```python
from build123d import *

# Parameters (mm, degrees)
SKETCH1_W              = 165.1
SKETCH1_H              = 114.3
BOSS_EXTRUDE1_DEPTH    = 6.35
F_10_24_TAPPED_HOLE2_D = 3.7973
F_6_32_TAPPED_HOLE2_D  = 2.7051
CUT_EXTRUDE10_DEPTH    = 101.602919938
F_6_32_TAPPED_HOLE1_D  = 2.7051
SKETCH24_W             = 107.95
SKETCH24_H             = 71.12
CUT_EXTRUDE11_DEPTH    = 101.602919938
FILLET1_R              = 3.175


with BuildPart() as part:
    # Sketch1 → Boss-Extrude1 (new body)
    with BuildSketch(Plane(origin=(0, 0, 0), x_dir=(1, 0, 0), z_dir=(0, 1, 0))):
        Rectangle(SKETCH1_W, SKETCH1_H)
    extrude(amount=BOSS_EXTRUDE1_DEPTH)

    # #10-24 Tapped Hole2 (through all)
    with Locations(Plane(origin=(0, 6.35, 0), x_dir=(-1, 0, 0), z_dir=(0, 1, 0))):
        with Locations((73.025, -47.625), (73.025, 47.625), (-73.025, -47.625), (-73.025, 47.625)):
            Hole(F_10_24_TAPPED_HOLE2_D / 2)

    # #6-32 Tapped Hole2 (through all)
    with Locations(Plane(origin=(0, 6.35, 0), x_dir=(-1, 0, 0), z_dir=(0, 1, 0))):
        with Locations((50.8, -44.45), (-50.8, -44.45), (-50.8, 44.45), (50.8, 44.45)):
            Hole(F_6_32_TAPPED_HOLE2_D / 2)

    # Sketch21 → Cut-Extrude10 (cut, through all)
    with BuildSketch(Plane(origin=(0, 6.35, 0), x_dir=(1, 0, 0), z_dir=(0, 1, 0))):
        with BuildLine():
            Line((-82.55, 20.94865), (-66.04, 20.94865))
            ThreePointArc((-66.04, 20.94865), (-64.14135, 19.05), (-66.04, 17.15135))
            Line((-66.04, 17.15135), (-82.55, 17.15135))
            ThreePointArc((-82.55, 17.15135), (-84.44865, 19.05), (-82.55, 20.94865))
        make_face()
        with BuildLine():
            Line((-82.55, -17.15135), (-66.04, -17.15135))
            ThreePointArc((-66.04, -17.15135), (-64.14135, -19.05), (-66.04, -20.94865))
            Line((-66.04, -20.94865), (-82.55, -20.94865))
            ThreePointArc((-82.55, -20.94865), (-84.44865, -19.05), (-82.55, -17.15135))
        make_face()
        with BuildLine():
            Line((-23.50135, 57.15), (-23.50135, 44.45))
            ThreePointArc((-23.50135, 44.45), (-25.4, 42.55135), (-27.29865, 44.45))
            Line((-27.29865, 44.45), (-27.29865, 57.15))
            ThreePointArc((-27.29865, 57.15), (-25.4, 59.04865), (-23.50135, 57.15))
        make_face()
        with BuildLine():
            Line((27.29865, 57.15), (27.29865, 44.45))
            ThreePointArc((27.29865, 44.45), (25.4, 42.55135), (23.50135, 44.45))
            Line((23.50135, 44.45), (23.50135, 57.15))
            ThreePointArc((23.50135, 57.15), (25.4, 59.04865), (27.29865, 57.15))
        make_face()
        with BuildLine():
            Line((66.04, 20.94865), (82.55, 20.94865))
            ThreePointArc((82.55, 20.94865), (84.44865, 19.05), (82.55, 17.15135))
            Line((82.55, 17.15135), (66.04, 17.15135))
            ThreePointArc((66.04, 17.15135), (64.14135, 19.05), (66.04, 20.94865))
        make_face()
        with BuildLine():
            Line((66.04, -17.15135), (82.55, -17.15135))
            ThreePointArc((82.55, -17.15135), (84.44865, -19.05), (82.55, -20.94865))
            Line((82.55, -20.94865), (66.04, -20.94865))
            ThreePointArc((66.04, -20.94865), (64.14135, -19.05), (66.04, -17.15135))
        make_face()
        with BuildLine():
            Line((-27.29865, -57.15), (-27.29865, -44.45))
            ThreePointArc((-27.29865, -44.45), (-25.4, -42.55135), (-23.50135, -44.45))
            Line((-23.50135, -44.45), (-23.50135, -57.15))
            ThreePointArc((-23.50135, -57.15), (-25.4, -59.04865), (-27.29865, -57.15))
        make_face()
        with BuildLine():
            Line((23.50135, -57.15), (23.50135, -44.45))
            ThreePointArc((23.50135, -44.45), (25.4, -42.55135), (27.29865, -44.45))
            Line((27.29865, -44.45), (27.29865, -57.15))
            ThreePointArc((27.29865, -57.15), (25.4, -59.04865), (23.50135, -57.15))
        make_face()
    extrude(amount=-CUT_EXTRUDE10_DEPTH, mode=Mode.SUBTRACT)

    # #6-32 Tapped Hole1 (through all)
    with Locations(Plane(origin=(0, 6.35, 0), x_dir=(-1, 0, 0), z_dir=(0, 1, 0))):
        with Locations((73.025, -38.1), (73.025, 38.1), (-73.025, -38.1), (-73.025, 38.1)):
            Hole(F_6_32_TAPPED_HOLE1_D / 2)

    # Sketch24 → Cut-Extrude11 (cut, through all)
    with BuildSketch(Plane(origin=(0, 6.35, 0), x_dir=(1, 0, 0), z_dir=(0, 1, 0))):
        Rectangle(SKETCH24_W, SKETCH24_H)
    extrude(amount=-CUT_EXTRUDE11_DEPTH, mode=Mode.SUBTRACT)

    # Fillet1
    fillet1_edges = [part.edges().sort_by_distance(p)[0] for p in [
        (-53.975, 3.175, 35.56),
        (-53.975, 3.175, -35.56),
        (53.975, 3.175, -35.56),
        (53.975, 3.175, 35.56),
    ]]
    fillet(fillet1_edges, radius=FILLET1_R)


solid = part.part
```
Geometry check sheet. Reference: the model listing, model coordinates, mm. A direction names the side the tool comes from. Give positions to 0.01 mm unless a question says otherwise; leave off trailing zeros. Loops run counter-clockwise (first coordinate to the right, second up) from the corner with the lowest first, then second, coordinate; pieces in that order, holes last. Notation, with made-up numbers: M -2,35 L 52,35 A26 cw 52,53 Z; hole C 81.5,29.5 d9. An arc over 180 degrees is marked long. Write item = value, one per line.
(1) Sectioned sample at A-A, the plane x = 25.4. Record the cut outline in (y, z), plus the area to 3 significant figures.
Answer below:
outline = M 0,-42.55 L 6.35,-42.55 L 6.35,-35.56 L 0,-35.56 Z; M 0,35.56 L 6.35,35.56 L 6.35,42.55 L 0,42.55 Z
area = 88.8 mm2
(2) Release check for a two-part mould opening along Z. For faces 1 (the face through (55, 3, 57.15)), 2 (the face through (-23.501, 3, 51)), 3 (the face through (55, 3, -57.15)), 4 (the face through (74, 3, 20.949)) record: released by +Z, released by -Z, zero draft, split by the parting line, or undercut.
Answer below:
face_1 = released by +Z
face_2 = zero draft
face_3 = released by -Z
face_4 = undercut
(3) Tool access check on faces 5 (the face through (-74, 3, -17.151)), 6 (the face through (53.975, 3, 0)), 7 (the face through (74, 3, 17.151)). Record the directions out of +Z, -Z, +X, -X, +Y, -Y that give a thin tool (end or side, any length) a straight path to the whole face; none if there is none.
Answer below:
face_5 = -X, +Y, -Y
face_6 = +Y, -Y
face_7 = +X, +Y, -Y
(4) Sectioned sample at C-C, the plane y = 3.25. State how many separate pieces and enclosed holes the cut face has, plus the area to 3 significant figures.
Answer below:
separate_pieces = 1
enclosed_holes = 13
area = 10,600 mm2
(5) Material ranges on line 1 (Z direction, x = -50.8, y = 2.75); line 2 (X direction, y = 2.5, z = 51); line 3 (Z direction, x = -12, y = 4.5), recorded low to high. Write a range as [from, to].
Answer below:
line_1 = [-57.15, -45.8], [-43.1, -35.56], [35.56, 43.1], [45.8, 57.15]
line_2 = [-82.55, -27.3], [-23.5, 23.5], [27.3, 82.55]
line_3 = [-57.15, -35.56], [35.56, 57.15]
(6) Sectioned sample at B-B, the plane z = -19.05. Record the cut outline in (x, y) (3 decimals), plus the area to 3 significant figures.
Answer below:
outline = M -64.141,0 L -53.975,0 L -53.975,6.35 L -64.141,6.35 Z; M 53.975,0 L 64.141,0 L 64.141,6.35 L 53.975,6.35 Z
area = 129 mm2
(7) Gauge pin test, flat ends, axial feed: pin 1 Ø3 at (x, z) = (73.025, 38.1) entering from -Y; pin 2 Ø2 at (x, z) = (-50.8, -44.45) entering from +Y; pin 3 Ø1 at (y, z) = (5, -18.5) entering from +X. Record the tip position at first contact, or that the pin passes through.
Answer below:
pin_1 = 0
pin_2 = through
pin_3 = 64.46
